```python
from build123d import *

# Parameters (mm, degrees)
F0_W     = 66.04
F0_H     = 25.4
F1_DEPTH = 17.78
F2_W     = 17.78
F2_H     = 25.4
F3_DEPTH = 25.4
F4_W     = 25.4
F4_H     = 25.4
F5_DEPTH = 50.8
F6_W     = 25.4
F6_H     = 25.4
F7_DEPTH = 25.4
F8_W     = 25.4
F8_H     = 25.4
F9_DEPTH = 68.58


with BuildPart() as f1:
    # F0 (on Right) → F1 (new body)
    with BuildSketch(Plane.YZ):
        with Locations((-37.761463, -42.327177)):
            Rectangle(F0_W, F0_H)
    extrude(amount=-F1_DEPTH)

    # F2 (on face) → F3 (join)
    with BuildSketch(Plane.XY.offset(-29.627177)):
        with Locations((-8.89, -17.441463)):
            Rectangle(F2_W, F2_H)
    extrude(amount=F3_DEPTH)

    # F4 (on face) → F5 (join)
    with BuildSketch(Plane(origin=(-17.78, 0, 0), x_dir=(0, -1, 0), z_dir=(-1, 0, 0))):
        with Locations((17.441463, -16.927177)):
            Rectangle(F4_W, F4_H)
    extrude(amount=F5_DEPTH)

    # F6 (on face) → F7 (join)
    with BuildSketch(Plane(origin=(0, 0, -29.627177), x_dir=(1, 0, 0), z_dir=(0, 0, -1))):
        with Locations((-55.88, 17.441463)):
            Rectangle(F6_W, F6_H)
    extrude(amount=F7_DEPTH)

    # F8 (on face) → F9 (join)
    with BuildSketch(Plane(origin=(0, -4.741463, 0), x_dir=(-1, 0, 0), z_dir=(0, 1, 0))):
        with Locations((55.88, -42.327177)):
            Rectangle(F8_W, F8_H)
    extrude(amount=F9_DEPTH)


solid = f1.part
```
Read the model definition and answer for the solid it produces. Units are mm, in the model's axes. A direction names the side the tool comes from. Coordinates: 2 decimals unless noted, no trailing zeros. Write each loop counter-clockwise with the first axis right and the second up, starting at its lowest first coordinate (ties: lowest second). Pieces come first, ordered by that corner, then holes. Notation, with made-up numbers: (9.5, -40) - (65.5, -40) arc R31 ccw to (65.5, -9) - close; hole circle Ø4 at (43, 34.5). An arc over 180 degrees is marked (long way). Answer as a JSON object with one key per item and string values. Group by question number.
1. Consider L1, parallel to X at y = -14.5, z = -50; L2, parallel to Y at x = -57, z = -46; L3, parallel to Z at x = -53, y = 10. Determine where each line is inside the solid, lowest interval first. Write a range as [from, to].
2. A cutting plane is placed at B-B (y = -27.5). Determine the outline of the cut face in (x, z), plus the area to 3 significant figures.
3. Which of the six approach directions +Z, -Z, +X, -X, +Y, -Y give full straight-line access (tool end or side, diameter ignored) to faces 1 (the flat face through (-30, -17, -29.627)), 2 (the flat face through (-9, -51, -29.627)), 3 (the flat face through (-27, -4.741, -24))?
4. The mould has two halves that part along X. Classify faces 4 (the flat face through (-43.18, 16, -43)), 5 (the flat face through (-9, -70.781, -43)), 6 (the flat face through (0, -31, -36)), 7 (the flat face through (-68.58, 6, -36)): +X half, -X half, draft (parallel to the pull), parting line (faces both ways), or undercut.
5. A cutting plane is placed at A-A (z = -44.5). Determine the outline of the cut face in (x, y), plus the area to 3 significant figures.
6. A cutting plane is placed at C-C (x = -54.5). Determine the outline of the cut face in (y, z).
7. Each of these flat-tipped pins is pushed along its axis until it touches: P1, Ø15, axis at x = -22, z = -22, coming from the -Y side; P2, Ø7.5, axis at y = 19.5, z = -46.5, coming from the +X side; P3, Ø7.5, axis at x = -33, y = -22, coming from the -Z side; P4, Ø3, axis at x = -41.5, y = 34.5, coming from the +Z side. Where does it stop, or does it pass through?
8. A cutting plane is placed at D-D (z = -7.5). Determine the outline of the cut face in (x, y), plus the area to 3 significant figures.
Worked out:
{
 "1": {"L1": "x = [-68.58, -43.18], [-17.78, 0]", "L2": "y = [-30.14, 63.84]", "L3": "z = [-55.03, -29.63]"},
 "2": {"outline": "(-68.58, -55.03) - (-43.18, -55.03) - (-43.18, -29.63) - (-17.78, -29.63) - (-17.78, -55.03) - (0, -55.03) - (0, -4.23) - (-68.58, -4.23) - close", "area": "2,840 mm²"},
 "3": {"face 1": "-Z, +Y, -Y", "face 2": "+Z, +X, -X, -Y", "face 3": "+Z, +X, +Y"},
 "4": {"face 4": "undercut", "face 5": "draft", "face 6": "+X half", "face 7": "-X half"},
 "5": {"outline": "(-68.58, -30.14) - (-43.18, -30.14) - (-43.18, 63.84) - (-68.58, 63.84) - close; (-17.78, -70.78) - (0, -70.78) - (0, -4.74) - (-17.78, -4.74) - close", "area": "3,560 mm²"},
 "6": {"outline": "(-30.14, -55.03) - (63.84, -55.03) - (63.84, -29.63) - (-4.74, -29.63) - (-4.74, -4.23) - (-30.14, -4.23) - close"},
 "7": {"P1": "stops at y = -30.14", "P2": "stops at x = -43.18", "P3": "stops at z = -29.63", "P4": "passes through"},
 "8": {"outline": "(-68.58, -30.14) - (0, -30.14) - (0, -4.74) - (-68.58, -4.74) - close", "area": "1,740 mm²"}
}
